from build123d import *

# Parameters (mm, degrees)
F0_W     = 152.4
F0_H     = 279.4
F1_DEPTH = 12.7


with BuildPart() as f1:
    # F0 (on Right) → F1 (new body)
    with BuildSketch(Plane.YZ):
        Rectangle(F0_W, F0_H)
        Polygon((-66.675, -52.705), (-70.485, -52.705), (-70.485, 125.095), (-70.485, 128.905), (-66.675, 128.905), (-60.325, 128.905), (-56.515, 128.905), (70.485, 128.905), (70.485, 125.095), (-56.515, 125.095), (-56.515, 112.395), (-56.515, -52.705), (-60.325, -52.705), (-60.325, -40.005), (-60.325, 112.395), (-60.325, 125.095), (-66.675, 125.095), align=None, mode=Mode.SUBTRACT)
    extrude(amount=-F1_DEPTH)


solid = f1.part
Can you work these out from the model? Positions are in its coordinate system, mm. A direction names the side the tool comes from. Round coordinates to 2 decimals unless told otherwise and drop trailing zeros. Loops run counter-clockwise (first coordinate to the right, second up) from the corner with the lowest first, then second, coordinate; pieces in that order, holes last. Notation, with made-up numbers: (-5, 64.5) - (23, 64.5) arc R30 ccw to (23, 97.5) - close; hole circle Ø11 at (-28.75, -19.75). An arc over 180 degrees is marked (long way). Write item = value, one per line. Start each with the question number.
(1) For faces 1 (the face through (-6, -60.325, 35)), 2 (the face through (-6, -1, 139.7)), which set-ups out of +Z, -Z, +X, -X, +Y, -Y let a thin tool reach every point of the face, with its end or its side?
(2) If we section it at A-A (z = 110): Please give me the cut outline in (x, y) (3 decimals), and give its area (3 significant figures).
(3) If we section it at B-B (x = -2.25): Please give me the cut outline in (y, z) (3 decimals), and give its area (3 significant figures).
(4) If I drill on probe 1 along Y at (x, z) = (-6, 58.5) (3 decimals); probe 2 along Z at (x, y) = (-4.25, 60) (3 decimals), over which ranges is the centre line in solid material (lowest first)? Write a range as [from, to].
(5) If we mould it in two halves opening along Y, with no side actions, what happens to faces 3 (the face through (-6, -76.2, -2)), 4 (the face through (-6, 76.2, -2)), 5 (the face through (-6, -63, 125.095)), 6 (the face through (-6, -70.485, 37))? For each: released by +Y, released by -Y, zero draft, split by the parting line, or undercut.
Ans:
q1.face_1 = +X, -X
q1.face_2 = +Z, +X, -X, +Y, -Y
q2.outline = (-12.7, -76.2) - (0, -76.2) - (0, -70.485) - (-12.7, -70.485) - close; (-12.7, -66.675) - (0, -66.675) - (0, -60.325) - (-12.7, -60.325) - close; (-12.7, -56.515) - (0, -56.515) - (0, 76.2) - (-12.7, 76.2) - close
q2.area = 1,840 mm²
q3.outline = (-76.2, -139.7) - (76.2, -139.7) - (76.2, 139.7) - (-76.2, 139.7) - close; hole (-70.485, -52.705) - (-66.675, -52.705) - (-66.675, 125.095) - (-60.325, 125.095) - (-60.325, -52.705) - (-56.515, -52.705) - (-56.515, 125.095) - (70.485, 125.095) - (70.485, 128.905) - (-70.485, 128.905) - close
q3.area = 40,700 mm²
q4.probe_1 = [-76.2, -70.485], [-66.675, -60.325], [-56.515, 76.2]
q4.probe_2 = [-139.7, 125.095], [128.905, 139.7]
q5.face_3 = released by -Y
q5.face_4 = released by +Y
q5.face_5 = undercut
q5.face_6 = undercut
